The figure shows three views and two pictorial views of one solid part (mm, origin at its lowest corner). Answer the questions. Give positions to 0.01 mm unless a question says otherwise; leave off trailing zeros. Write each loop counter-clockwise with the first axis right and the second up, starting at its lowest first coordinate (ties: lowest second). Pieces come first, ordered by that corner, then holes. Notation, with made-up numbers: M 56.5,7 L 108.5,7 A21 cw 108.5,16 Z; hole C 75.25,53.5 d2. An arc over 180 degrees is marked long. Answer as CSV lines item,"result". Start each with the question number.
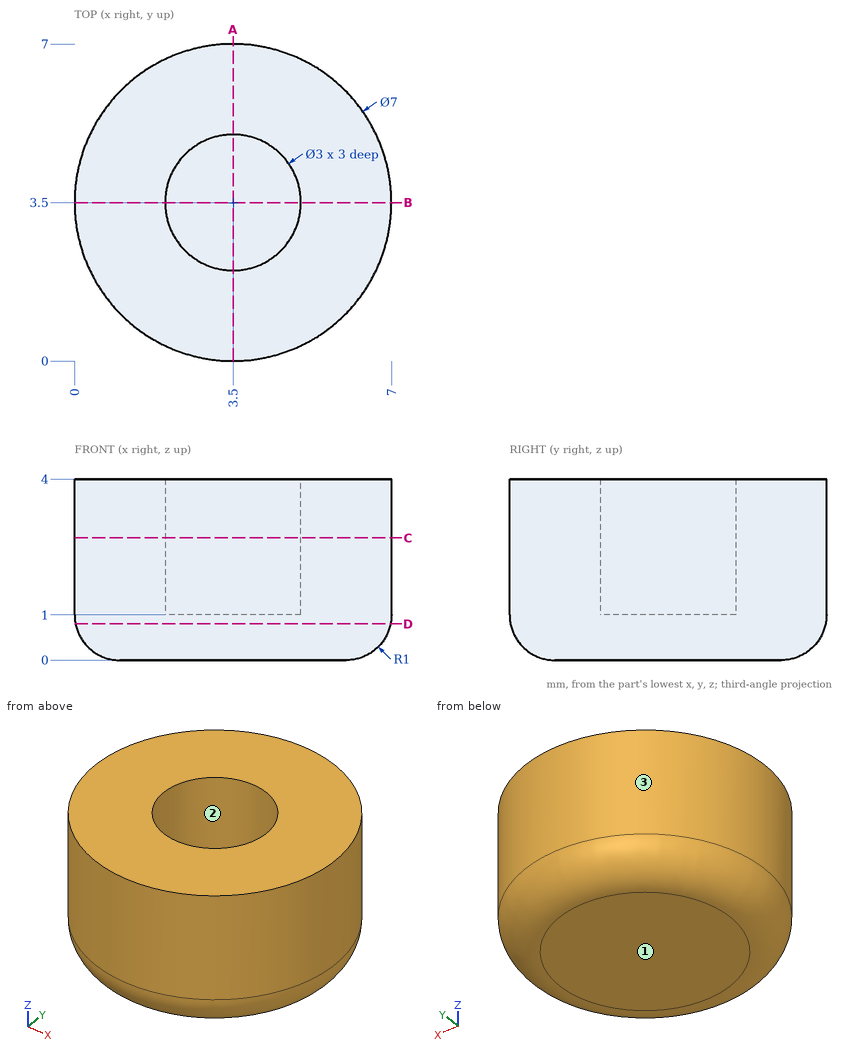
1. Given pin 1 (4 mm diameter, centred on x = 3.5, y = 3.5, fed in from +Z); pin 2 (1.5 mm diameter, centred on x = 3, y = 4, fed in from +Z), each flat-ended and moving along its own axis, determine where each tip first touches the part or whether it passes through.
2. Find section D-D on z = 0.8. Determine the outline of the cut face in (x, y).
3. Find section A-A on x = 3.5. Determine the outline of the cut face in (y, z).
4. Determine the mould class of the marked faces 1, 2 and 3 for opening direction Y: +Y half, -Y half, draft (parallel to the pull), parting line (faces both ways), or undercut.
5. Find section C-C on z = 2.7. Determine the outline of the cut face in (x, y), then the cut area to 3 significant figures.
6. Find the intervals of material crossed by line 1 (Y direction, x = 3.5, z = 1.7); line 2 (Z direction, x = 1, y = 3); line 3 (Y direction, x = 2.5, z = 1.8), in increasing order. Write a range as [from, to].
Computed:
1,pin 1,"stops at z = 4"
1,pin 2,"stops at z = 1"
2,outline,"C 3.5,3.5 d6.96"
3,outline,"M 0,1 A1 ccw 1,0 L 6,0 A1 ccw 7,1 L 7,4 L 5,4 L 5,1 L 2,1 L 2,4 L 0,4 Z"
4,face 1,"draft"
4,face 2,"undercut"
4,face 3,"parting line"
5,outline,"C 3.5,3.5 d7; hole C 3.5,3.5 d3"
5,area,"31.4 mm^2"
6,line 1,"y = [0, 2], [5, 7]"
6,line 2,"z = [0, 4]"
6,line 3,"y = [0.15, 2.38], [4.62, 6.85]"
